from build123d import *

# Parameters (mm, degrees)
F1_DEPTH = 609.6
F2_R     = 2.4765
F3_DEPTH = 50.801


with BuildPart() as f1:
    # F0 (on Top) → F1 (new body)
    with BuildSketch(Plane.XY):
        Polygon((0, 0), (0, 47.625), (-3.175, 47.625), (-3.175, -3.175), (22.225, -3.175), (22.225, 0), align=None)
    extrude(amount=F1_DEPTH)

    # F2 (on face) → F3 (cut, through all)
    with BuildSketch(Plane.XZ.offset(3.175)):
        with Locations((9.525, 12.7)):
            Circle(F2_R)
        with Locations((9.525, 190.5)):
            Circle(F2_R)
        with Locations((9.525, 419.1)):
            Circle(F2_R)
        with Locations((9.525, 596.9)):
            Circle(F2_R)
    extrude(amount=-F3_DEPTH, mode=Mode.SUBTRACT)


solid = f1.part
For this review, take the finished solid that the model builds, in its own axes (mm). A direction names the side the tool comes from. Round coordinates to 2 decimals unless told otherwise and drop trailing zeros. Order: outer loops, then holes, each group sorted by start corner. A loop starts at its lowest first (then second) coordinate and runs counter-clockwise, first axis right, second up. Notation, with made-up numbers: M -35,13 L -28,13 A26 ccw -28,34 Z; hole C -3,43.5 d7. An arc over 180 degrees is marked long. Use a Markdown table: item, result. Add a question column.
Item 1: Add section B-B, the plane y = 34. Give the boundary of the cut face in (x, z) (3 decimals), then the cut area to 3 significant figures.
Item 2: To check wall thickness, follow line 1 along X through (y, z) = (-1.2, 190.5) (1 decimal); line 2 along X through (y, z) = (-2, 419) (3 decimals); line 3 along Y through (x, z) = (20.5, 385) (3 decimals). State the ranges of each line that lie inside material, in increasing order.
Item 3: Add section A-A, the plane z = 505.5. Give the boundary of the cut face in (x, y) (3 decimals), then the cut area to 3 significant figures.
Item 4: Tool access review of faces 1 (the flat face through (11, 0, 301)), 2 (the flat face through (9, -3.175, 301)): name each direction out of +Z, -Z, +X, -X, +Y, -Y from which nothing blocks a thin tool from reaching the whole face with its end or side.
Item 5: Insertion check: pin 1 (8 mm diameter, centred on y = 18.5, z = 510, fed in from +X); pin 2 (4 mm diameter, centred on x = 9.525, z = 419.1, fed in from +Y); pin 3 (3 mm diameter, centred on x = 2.5, z = 536, fed in from +Y). Each pin has a flat end and moves straight along its axis. Give the tip position at first contact, or say it passes through.
Geometry results:
| question | item | result |
|---|---|---|
| 1 | outline | M -3.175,0 L 0,0 L 0,609.6 L -3.175,609.6 Z |
| 1 | area | 1,940 mm² |
| 2 | line 1 | x = -3.2 to 7, 12 to 22.2 |
| 2 | line 2 | x = -3.175 to 7.051, 11.999 to 22.225 |
| 2 | line 3 | y = -3.175 to 0 |
| 3 | outline | M -3.175,-3.175 L 22.225,-3.175 L 22.225,0 L 0,0 L 0,47.625 L -3.175,47.625 Z |
| 3 | area | 232 mm² |
| 4 | face 1 | +Z, -Z, +X, +Y |
| 4 | face 2 | +Z, -Z, +X, -X, -Y |
| 5 | pin 1 | stops at x = 0 |
| 5 | pin 2 | passes through |
| 5 | pin 3 | stops at y = 0 |
